Geometry check sheet. Reference: the model listing, model coordinates, mm. A direction names the side the tool comes from. Coordinates: 2 decimals unless noted, no trailing zeros. Write each loop counter-clockwise with the first axis right and the second up, starting at its lowest first coordinate (ties: lowest second). Pieces come first, ordered by that corner, then holes. Notation, with made-up numbers: (74.25, 88) -> (105.25, 88) arc R27 ccw to (105.25, 111) -> close; hole circle Ø9 at (-16, 31). An arc over 180 degrees is marked (long way). Answer in a Markdown table with one row per item. Add a question column.
Q1. Gauge pin test, flat ends, axial feed: P1, Ø3, axis at x = 0, z = 0, coming from the -Y side; P2, Ø1.5, axis at x = -18.5, z = -16.5, coming from the +Y side; P3, Ø2, axis at x = 0, z = -39.03, coming from the -Y side. Record the tip position at first contact, or that the pin passes through.
Q2. Thickness scan on line 1 (Z direction, x = 0, y = -28.2); line 2 (Z direction, x = -37.5, y = -5); line 3 (X direction, y = -6, z = -25). Record the ranges inside material, lowest first.
Q3. Section check A-A, the plane y = -21. Record the boundary of the cut face in (x, z), and give its area (3 significant figures).
Q4. Section check D-D, the plane z = -47. Record the boundary of the cut face in (x, y).
Q5. Section check C-C, the plane z = 0. Record the boundary of the cut face in (x, y), and give its area (3 significant figures).
Q6. Tool access check on faces 5 (the face through (54.889, -12, -1)), 6 (the face through (-1, -32, 52.019)), 7 (the face through (-40, -27, -1)). Record the directions out of +Z, -Z, +X, -X, +Y, -Y that give a thin tool (end or side, any length) a straight path to the whole face; none if there is none.
Q7. Section check B-B, the plane x = 0. Record the boundary of the cut face in (y, z), and give its area (3 significant figures).
Q8. Release check for a two-part mould opening along Z. For faces 1 (the face through (-1, -17, 55.076)), 2 (the face through (55.811, -32, -1)), 3 (the face through (59.889, -17, -1)), 4 (the face through (40.42, -27.47, 0.06)) record: pulls with the +Z half, pulls with the -Z half, needs draft (parallel to the pull), parting line crosses it, or undercut.
```python
from build123d import *

# Parameters (mm, degrees)
F0_W     = 120
F0_H     = 110
F0_W_2   = 110
F0_H_2   = 100
F1_DEPTH = 25
F2_W     = 120
F2_H     = 110
F2_W_2   = 110
F2_H_2   = 100
F3_DEPTH = 5
F4_W     = 120
F4_H     = 110
F4_W_2   = 112.4888285995
F4_H_2   = 103.6703959107
F5_DEPTH = 5
F7_D     = 2.794


with BuildPart() as f1:
    # F0 (on Front) → F1 (new body)
    with BuildSketch(Plane.XZ):
        with Locations((-0.1109875739, 0.0762201769)):
            Rectangle(F0_W, F0_H)
        with Locations((-0.1109875739, -0.0193089247)):
            Rectangle(F0_W_2, F0_H_2, mode=Mode.SUBTRACT)
    extrude(amount=F1_DEPTH)

    # F2 (on face) → F3 (join)
    with BuildSketch(Plane.XZ.offset(25)):
        with Locations((-0.1109875739, 0.0762201769)):
            Rectangle(F2_W, F2_H)
        with Locations((-0.1109875739, -0.0193089247)):
            Rectangle(F2_W_2, F2_H_2, mode=Mode.SUBTRACT)
        with Locations((-0.1109875739, -0.0193089247)):
            Rectangle(F2_W_2, F2_H_2)
    extrude(amount=F3_DEPTH)

    # F4 (on face) → F5 (join)
    with BuildSketch(Plane.XZ.offset(30)):
        with Locations((-0.1109875739, 0.0762201769)):
            Rectangle(F4_W, F4_H)
        with Locations((-0.4336126149, 0.1837611198)):
            Rectangle(F4_W_2, F4_H_2, mode=Mode.SUBTRACT)
    extrude(amount=F5_DEPTH)

    # F7 (through all)
    with Locations(Plane.XZ.offset(30)):
        with Locations((0, 39.025651645), (-39.025651645, 0), (0, -39.025651645), (39.025651645, 0), (0, 0)):
            Hole(F7_D / 2)


solid = f1.part
```
Calculated:
| question | item | result |
|---|---|---|
| 1 | P1 | stops at y = -30 |
| 1 | P2 | stops at y = -25 |
| 1 | P3 | passes through |
| 2 | line 1 | z = -54.92 to -40.42, -37.63 to -1.4, 1.4 to 37.63, 40.42 to 55.08 |
| 2 | line 2 | z = -54.92 to -50.02, 49.98 to 55.08 |
| 2 | line 3 | x = -60.11 to -55.11, 54.89 to 59.89 |
| 3 | outline | (-60.11, -54.92) -> (59.89, -54.92) -> (59.89, 55.08) -> (-60.11, 55.08) -> close; hole (-55.11, -50.02) -> (54.89, -50.02) -> (54.89, 49.98) -> (-55.11, 49.98) -> close |
| 3 | area | 2,200 mm² |
| 4 | outline | (-60.11, -35) -> (-56.68, -35) -> (-56.68, -30) -> (55.81, -30) -> (55.81, -35) -> (59.89, -35) -> (59.89, 0) -> (54.89, 0) -> (54.89, -25) -> (-55.11, -25) -> (-55.11, 0) -> (-60.11, 0) -> close |
| 5 | outline | (-60.11, -35) -> (-56.68, -35) -> (-56.68, -30) -> (-40.42, -30) -> (-40.42, -25) -> (-55.11, -25) -> (-55.11, 0) -> (-60.11, 0) -> close; (-37.63, -30) -> (-1.4, -30) -> (-1.4, -25) -> (-37.63, -25) -> close; (1.4, -30) -> (37.63, -30) -> (37.63, -25) -> (1.4, -25) -> close; (40.42, -30) -> (55.81, -30) -> (55.81, -35) -> (59.89, -35) -> (59.89, 0) -> (54.89, 0) -> (54.89, -25) -> (40.42, -25) -> close |
| 5 | area | 846 mm² |
| 6 | face 5 | +Y |
| 6 | face 6 | -Y |
| 6 | face 7 | +Y, -Y |
| 7 | outline | (-35, -54.92) -> (0, -54.92) -> (0, -50.02) -> (-25, -50.02) -> (-25, -40.42) -> (-30, -40.42) -> (-30, -51.65) -> (-35, -51.65) -> close; (-35, 52.02) -> (-30, 52.02) -> (-30, 40.42) -> (-25, 40.42) -> (-25, 49.98) -> (0, 49.98) -> (0, 55.08) -> (-35, 55.08) -> close; (-30, -37.63) -> (-25, -37.63) -> (-25, -1.4) -> (-30, -1.4) -> close; (-30, 1.4) -> (-25, 1.4) -> (-25, 37.63) -> (-30, 37.63) -> close |
| 7 | area | 790 mm² |
| 8 | face 1 | pulls with the +Z half |
| 8 | face 2 | undercut |
| 8 | face 3 | needs draft |
| 8 | face 4 | undercut |
